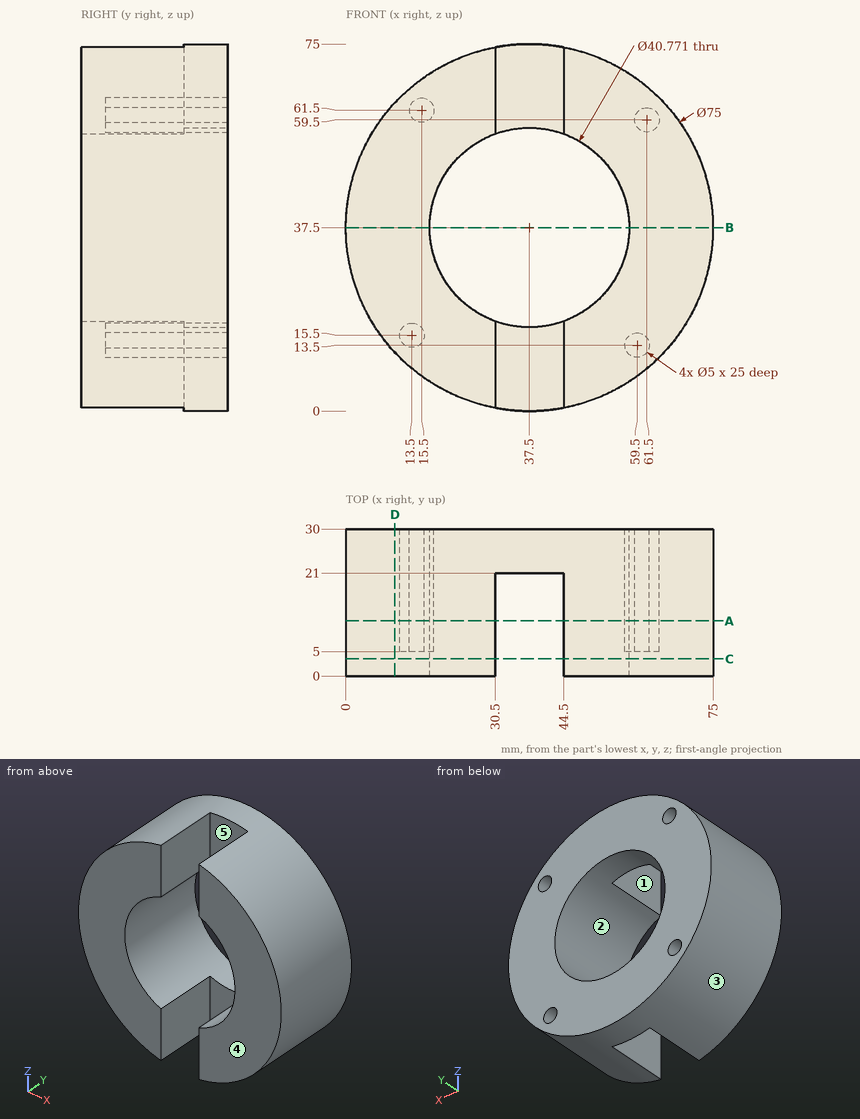
Design review of the part shown in the three views and the two pictorial views. Dimensions are in mm from the part's minimum x, y and z. A direction names the side the tool comes from. Round coordinates to 2 decimals unless told otherwise and drop trailing zeros. Write each loop counter-clockwise with the first axis right and the second up, starting at its lowest first coordinate (ties: lowest second). Pieces come first, ordered by that corner, then holes. Notation, with made-up numbers: M 84,26 L 141,26 A28 cw 141,64 Z; hole C 64,-21 d6. An arc over 180 degrees is marked long. Use a Markdown table: item, result. Add a question column.
Q1. We need section D-D, the plane x = 10. State the section outline as (y, z) points (3 decimals).
Q2. Machinability: for the marked faces 4 and 5, which of the approach directions +Z, -Z, +X, -X, +Y, -Y give a long, thin tool a straight path to every point of the face, cutting with its end or side? Answer none if there is none.
Q3. To check wall thickness, follow line 1 (X direction, y = 14, z = 59.5); line 2 (X direction, y = 9.5, z = 37.5); line 3 (Z direction, x = 50, y = 17) (1 decimal). State the ranges of each line that lie inside material, in increasing order.
Q4. Insertion check: pin 1 (6 mm diameter, centred on y = 16, z = 53.5, fed in from +X); pin 2 (5.5 mm diameter, centred on y = 13, z = 61.5, fed in from -X); pin 3 (14 mm diameter, centred on y = 12, z = 6.5, fed in from +X). Each pin has a flat end and moves straight along its axis. Give the tip position at first contact, or say it passes through.
Q5. We need section C-C, the plane y = 3.5. State the section outline as (x, z) points.
Q6. We need section A-A, the plane y = 11.25. State the section outline as (x, z) points, plus the area to 3 significant figures.
Q7. The part is to be moulded in two halves that separate along Z. For the marked faces 1, 2 and 3, say which applies: pulls with the +Z half, pulls with the -Z half, needs draft (parallel to the pull), parting line crosses it, or undercut.
Q8. We need section B-B, the plane z = 37.5. State the section outline as (x, y) points, plus the area to 3 significant figures.
Findings below:
| question | item | result |
|---|---|---|
| 1 | outline | M 0,12.005 L 30,12.005 L 30,62.995 L 0,62.995 Z |
| 2 | face 4 | +Z, -Z, +X, -X, -Y |
| 2 | face 5 | +Z, -Z, -Y |
| 3 | line 1 | x = 7.13 to 14, 17 to 30.5, 44.5 to 59, 64 to 67.87 |
| 3 | line 2 | x = 0 to 17.11, 57.89 to 75 |
| 3 | line 3 | z = 2.1 to 21.4, 53.6 to 72.9 |
| 4 | pin 1 | stops at x = 72.67 |
| 4 | pin 2 | stops at x = 6.6 |
| 4 | pin 3 | stops at x = 66.31 |
| 5 | outline | M 30.5,0.66 L 30.5,18.35 A20.39 cw 30.5,56.65 L 30.5,74.34 A37.5 ccw Z; M 44.5,0.66 A37.5 ccw 44.5,74.34 L 44.5,56.65 A20.39 cw 44.5,18.35 Z |
| 6 | outline | M 30.5,0.66 L 30.5,18.35 A20.39 cw 30.5,56.65 L 30.5,74.34 A37.5 ccw Z; M 44.5,0.66 A37.5 ccw 44.5,74.34 L 44.5,56.65 A20.39 cw 44.5,18.35 Z; hole C 13.5,15.5 d5; hole C 15.5,61.5 d5; hole C 59.5,13.5 d5; hole C 61.5,59.5 d5 |
| 6 | area | 2,550 mm² |
| 7 | face 1 | needs draft |
| 7 | face 2 | undercut |
| 7 | face 3 | parting line crosses it |
| 8 | outline | M 0,0 L 17.11,0 L 17.11,30 L 0,30 Z; M 57.89,0 L 75,0 L 75,30 L 57.89,30 Z |
| 8 | area | 1,030 mm² |
